```python
from build123d import *

# Parameters (mm, degrees)
SKETCH1_W               = 10
SKETCH1_H               = 29
BOSS_EXTRUDE1_DEPTH     = 34
CUT_EXTRUDE1_DEPTH      = 45.55333882
CUT_EXTRUDE1_DEPTH_BACK = 45.55333882
SKETCH2_R               = 11.9
FILLET1_R               = 1
FILLET2_R               = 7
CUT_EXTRUDE2_DEPTH      = 45.55333882
CUT_EXTRUDE2_DEPTH_BACK = 45.55333882
FILLET3_R               = 1
FILLET4_R               = 1
FILLET5_R               = 7


with BuildPart() as part:
    # Sketch1 → Boss-Extrude1 (new body)
    with BuildSketch(Plane.XY):
        with Locations((5, 12.5)):
            Rectangle(SKETCH1_W, SKETCH1_H)
    extrude(amount=BOSS_EXTRUDE1_DEPTH)

    # Sketch2 → Cut-Extrude1 (cut, two sides: drawn at the far end of the back side and taken through both)
    with BuildSketch(Plane(origin=(10, 0, 0), x_dir=(0, 0, -1), z_dir=(1, 0, 0)).offset(-CUT_EXTRUDE1_DEPTH_BACK)):
        with Locations((-15, 12.5)):
            Circle(SKETCH2_R)
    extrude(amount=CUT_EXTRUDE1_DEPTH + CUT_EXTRUDE1_DEPTH_BACK, mode=Mode.SUBTRACT)

    # Fillet1
    fillet1_edges = [part.edges().sort_by_distance(p)[0] for p in [
        (0, 12.5, 26.9),
        (10, 12.5, 26.9),
    ]]
    fillet(fillet1_edges, radius=FILLET1_R)

    # Fillet2
    fillet2_edges = [part.edges().sort_by_distance(p)[0] for p in [
        (5, 27, 0),
        (5, -2, 0),
    ]]
    fillet(fillet2_edges, radius=FILLET2_R)

    # Sketch3 → Cut-Extrude2 (cut, two sides: drawn at the far end of the back side and taken through both)
    with BuildSketch(Plane(origin=(10, 0, 0), x_dir=(0, 0, -1), z_dir=(1, 0, 0)).offset(-CUT_EXTRUDE2_DEPTH_BACK)):
        Polygon((-29.5, 12.5), (-29.5, 16.5), (-30.5, 16.5), (-30.5, 8.5), (-29.5, 8.5), align=None)
    extrude(amount=CUT_EXTRUDE2_DEPTH + CUT_EXTRUDE2_DEPTH_BACK, mode=Mode.SUBTRACT)

    # Fillet3
    fillet3_edges = [part.edges().sort_by_distance(p)[0] for p in [
        (0, 8.5, 30),
        (0, 12.5, 30.5),
        (0, 16.5, 30),
        (0, 12.5, 29.5),
    ]]
    fillet(fillet3_edges, radius=FILLET3_R)

    # Fillet4
    fillet4_edges = [part.edges().sort_by_distance(p)[0] for p in [
        (10, 12.5, 29.5),
        (10, 16.5, 30),
        (10, 12.5, 30.5),
        (10, 8.5, 30),
    ]]
    fillet(fillet4_edges, radius=FILLET4_R)

    # Fillet5
    fillet5_edges = [part.edges().sort_by_distance(p)[0] for p in [
        (5, 27, 34),
        (5, -2, 34),
    ]]
    fillet(fillet5_edges, radius=FILLET5_R)


solid = part.part
```
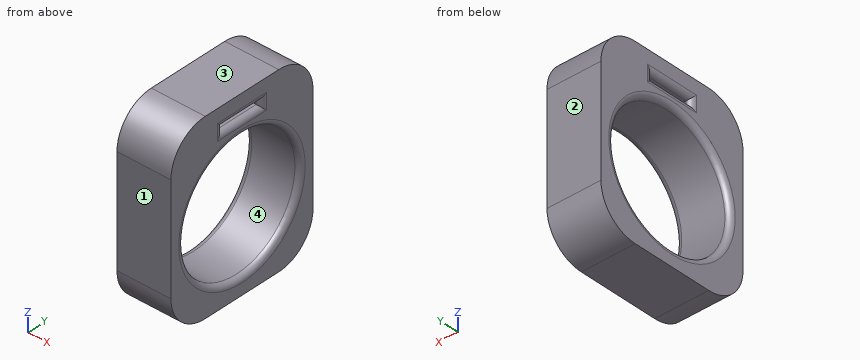
Check sheet for the modelled part. Datum: model origin and axes. Units: mm. Face numbers are marked on the shaded views. Coordinates: 2 decimals unless noted, no trailing zeros. Loops run counter-clockwise (first coordinate to the right, second up) from the corner with the lowest first, then second, coordinate; pieces in that order, holes last.
1) Sectioned sample at C-C (y = 12.5). Record the boundary of the cut face in (x, z).
2) Sectioned sample at A-A (z = 15). Record the boundary of the cut face in (x, y), and give its area (3 significant figures).
3) Release check for a two-part mould opening along Y. For the marked faces 1, 2, 3 and 4 record: released by +Y, released by -Y, zero draft, split by the parting line, or undercut.
4) Sectioned sample at B-B (x = 5). Record the boundary of the cut face in (y, z).
5) Gauge pin test, flat ends, axial feed: pin 1 (0.5 mm diameter, centred on x = 7, z = 30, fed in from -Y); pin 2 (0.5 mm diameter, centred on x = 6, z = 30, fed in from +Y); pin 3 (4 mm diameter, centred on x = 7.5, z = 29.5, fed in from -Y). Record the tip position at first contact, or that the pin passes through.
6) Material ranges on probe 1 along Z at (x, y) = (3.5, 12.5); probe 2 along Y at (x, z) = (4, 15); probe 3 along Z at (x, y) = (2.75, 10.5), recorded low to high.
Check sheet entries:
1. outline: (0, 0) - (10, 0) - (10, 2.1) arc R1 ccw to (9, 3.1) - (1, 3.1) arc R1 ccw to (0, 2.1) - close; (0, 27.9) arc R1 ccw to (1, 26.9) - (9, 26.9) arc R1 ccw to (10, 27.9) - (10, 28.5) arc R1 ccw to (9, 29.5) - (1, 29.5) arc R1 ccw to (0, 28.5) - close; (0, 31.5) arc R1 ccw to (1, 30.5) - (9, 30.5) arc R1 ccw to (10, 31.5) - (10, 34) - (0, 34) - close
2. outline: (0, -2) - (10, -2) - (10, -0.4) arc R1 ccw to (9, 0.6) - (1, 0.6) arc R1 ccw to (0, -0.4) - close; (0, 25.4) arc R1 ccw to (1, 24.4) - (9, 24.4) arc R1 ccw to (10, 25.4) - (10, 27) - (0, 27) - close
2. area: 51.1 mm2
3. face 1: released by -Y
3. face 2: released by +Y
3. face 3: zero draft
3. face 4: undercut
4. outline: (-2, 7) arc R7 ccw to (5, 0) - (20, 0) arc R7 ccw to (27, 7) - (27, 27) arc R7 ccw to (20, 34) - (5, 34) arc R7 ccw to (-2, 27) - close; hole circle Ø23.8 at (12.5, 15); hole (8.5, 29.5) - (16.5, 29.5) - (16.5, 30.5) - (8.5, 30.5) - close
5. pin 1: stops at y = -1.44
5. pin 2: stops at y = 26.44
5. pin 3: stops at y = -1.98
6. probe 1: z = 0 to 3.1, 26.9 to 29.5, 30.5 to 34
6. probe 2: y = -2 to 0.6, 24.4 to 27
6. probe 3: z = 0 to 3.27, 26.73 to 29.5, 30.5 to 34
